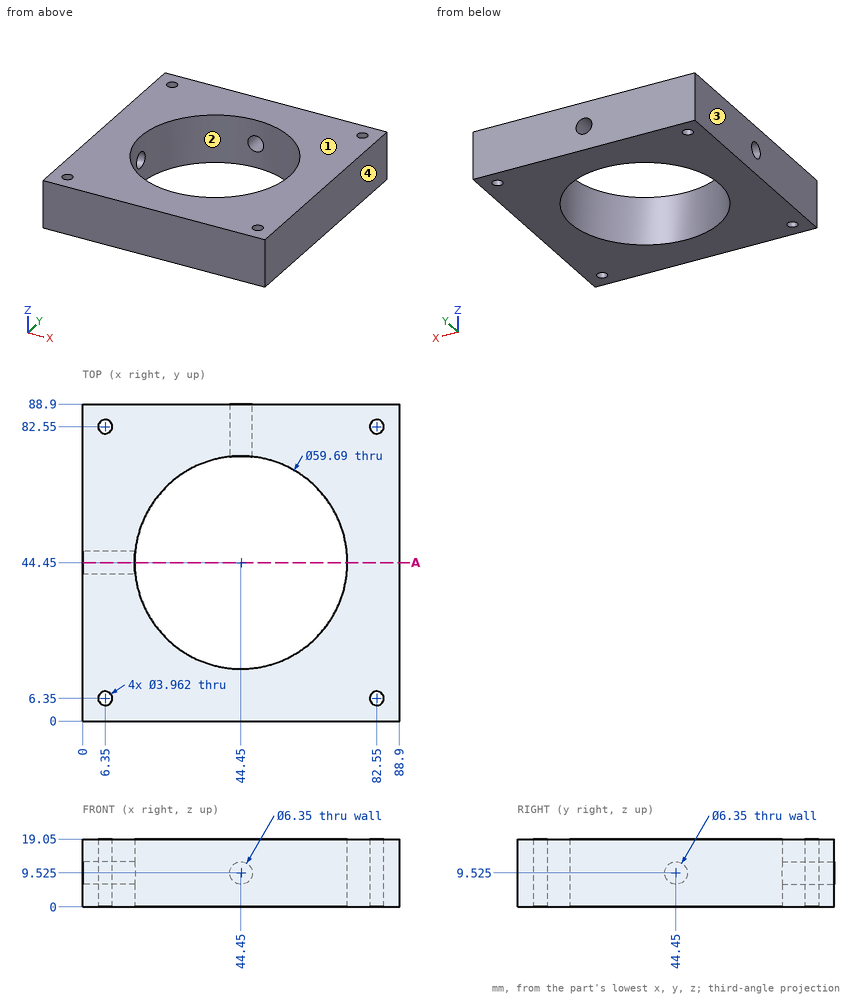
Study the drawing (mm; zero at the part's minimum x, y, z) and answer. Give positions to 0.01 mm unless a question says otherwise; leave off trailing zeros. Write item = value, one per line. Start each with the question number.
(1) The mould has two halves that part along X. Classify the marked faces 1, 2, 3 and 4: +X half, -X half, draft (parallel to the pull), parting line (faces both ways), or undercut.
(2) Find section A-A on y = 44.45. Give the number of separate pieces and of enclosed holes in the cut face, and give its area (3 significant figures).
(3) Find the intervals of material crossed by probe 1 along X at (y, z) = (82.5, 2.5); probe 2 along X at (y, z) = (81, 10.75) (1 decimal), in increasing order. Write a range as from..to.
(4) Given pin 1 Ø2.5 at (x, y) = (6.35, 82.55) entering from +Z, flat-ended and moving along its own axis, determine where the tip first touches the part or whether it passes through.
From the geometry:
q1.face_1 = draft
q1.face_2 = undercut
q1.face_3 = -X half
q1.face_4 = +X half
q2.separate_pieces = 3
q2.enclosed_holes = 0
q2.area = 464 mm^2
q3.probe_1 = 0..4.37, 8.33..80.57, 84.53..88.9
q3.probe_2 = 0..5.1, 7.6..41.5, 47.4..81.3, 83.8..88.9
q4.pin_1 = through
